For this review, use the dimensioned drawing (mm, ordinates from the lowest corner) and the shaded views. A direction names the side the tool comes from. Coordinates: 2 decimals unless noted, no trailing zeros. Loops run counter-clockwise (first coordinate to the right, second up) from the corner with the lowest first, then second, coordinate; pieces in that order, holes last. Notation, with made-up numbers: (-2, -11.75) - (10, -11.75) arc R22 ccw to (10, 5.25) - close; hole circle Ø6 at (-40, 38.5). An arc over 180 degrees is marked (long way). Return JSON: item names as keys, results as strings. Group by question number.
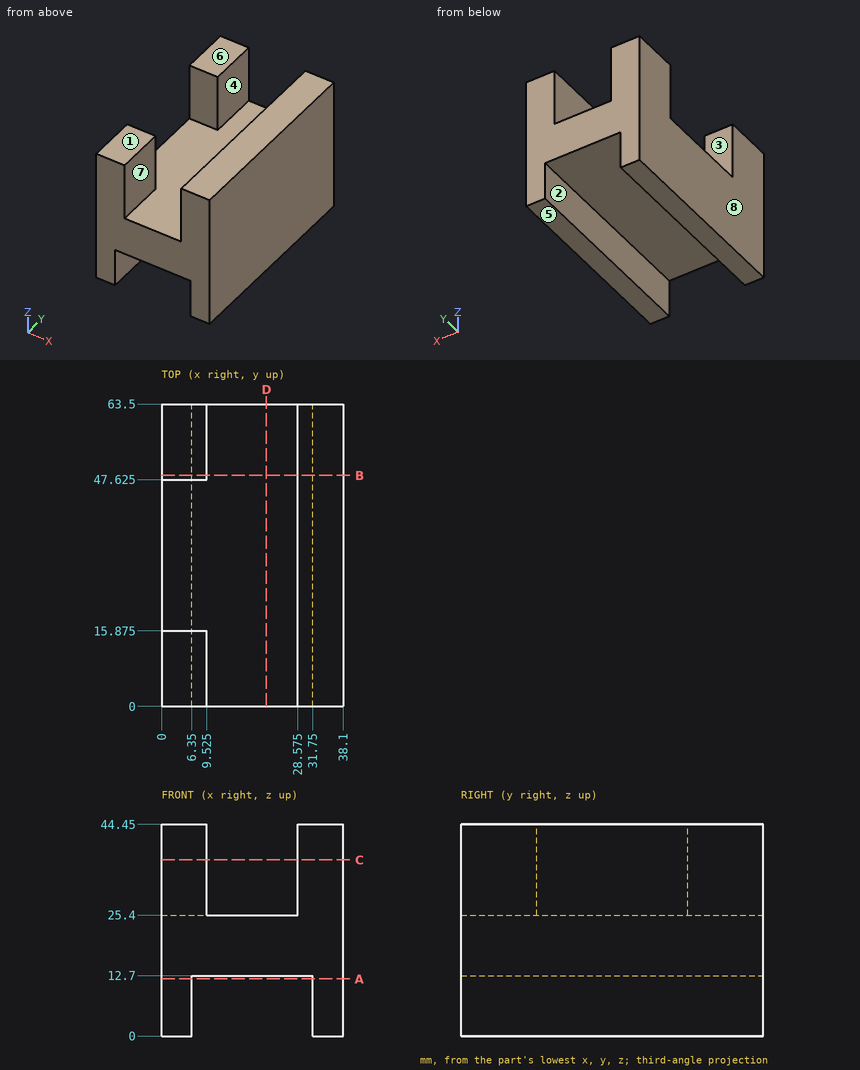
Item 1: For the marked faces 1, 2, 3, 4 and 5, list the 3-axis set-ups (+Z, -Z, +X, -X, +Y, -Y) from which the entire face can be reached by the end or side of a thin tool; tool diameter is ignored.
Item 2: For P1, Ø1, axis at x = 8.5, z = 5, coming from the +Y side; P2, Ø7.5, axis at x = 13, y = 26.5, coming from the -Z side; P3, Ø4, axis at x = 23, y = 54.5, coming from the +Z side, all flat-tipped, find the tip position at first contact; note any pin that passes through.
Item 3: Add section D-D (x = 22). State the section outline as (y, z) points.
Item 4: Add section A-A (z = 12). State the section outline as (x, y) points, then the cut area to 3 significant figures.
Item 5: To check wall thickness, follow line 1 (X direction, y = 5, z = 7); line 2 (X direction, y = 57, z = 26) (3 decimals); line 3 (Z direction, x = 20, y = 21). State the ranges of each line that lie inside material, in increasing order. Write a range as from..to.
Item 6: Add section C-C (z = 37). State the section outline as (x, y) points (3 decimals).
Item 7: Add section B-B (y = 48.5). State the section outline as (x, z) points (3 decimals), then the cut area to 3 significant figures.
Item 8: Draft analysis for pull direction X (two halves, no side actions). For the marked faces 6, 7 and 8, state which applies: pulls with the +X half, pulls with the -X half, needs draft (parallel to the pull), parting line crosses it, or undercut.
Answers below:
{
 "1": {"face 1": "+Z, +X, -X, +Y, -Y", "face 2": "-Z, +Y, -Y", "face 3": "+Z, -X", "face 4": "+Z, +Y, -Y", "face 5": "-Z, +X, -X, +Y, -Y"},
 "2": {"P1": "passes through", "P2": "stops at z = 12.7", "P3": "stops at z = 25.4"},
 "3": {"outline": "(0, 12.7) - (63.5, 12.7) - (63.5, 25.4) - (0, 25.4) - close"},
 "4": {"outline": "(0, 0) - (6.35, 0) - (6.35, 63.5) - (0, 63.5) - close; (31.75, 0) - (38.1, 0) - (38.1, 63.5) - (31.75, 63.5) - close", "area": "806 mm^2"},
 "5": {"line 1": "x = 0..6.35, 31.75..38.1", "line 2": "x = 0..9.525, 28.575..38.1", "line 3": "z = 12.7..25.4"},
 "6": {"outline": "(0, 0) - (9.525, 0) - (9.525, 15.875) - (0, 15.875) - close; (0, 47.625) - (9.525, 47.625) - (9.525, 63.5) - (0, 63.5) - close; (28.575, 0) - (38.1, 0) - (38.1, 63.5) - (28.575, 63.5) - close"},
 "7": {"outline": "(0, 0) - (6.35, 0) - (6.35, 12.7) - (31.75, 12.7) - (31.75, 0) - (38.1, 0) - (38.1, 44.45) - (28.575, 44.45) - (28.575, 25.4) - (9.525, 25.4) - (9.525, 44.45) - (0, 44.45) - close", "area": "1,010 mm^2"},
 "8": {"face 6": "needs draft", "face 7": "undercut", "face 8": "pulls with the -X half"}
}
